Model file for the job. Use its own axes, mm. Coordinates: 2 decimals unless noted, no trailing zeros. Order: outer loops, then holes, each group sorted by start corner. A loop starts at its lowest first (then second) coordinate and runs counter-clockwise, first axis right, second up. Notation, with made-up numbers: (-2.5, 47) - (31.5, 47) arc R37 ccw to (31.5, 83) - close; hole circle Ø7 at (-30.5, -31.5). An arc over 180 degrees is marked (long way). Put each result on its own line as item: value. Start each with the question number.
```python
from build123d import *

# Parameters (mm, degrees)
F0_W     = 60
F0_H     = 60
F1_DEPTH = 10
F2_R     = 4.99999


# Not quite as in the source:
# - a fillet or chamfer is up to 0.001 mm smaller than in the source, because OpenCascade refuses the exact size


with BuildPart() as f1:
    # F0 (on Top) → F1 (new body)
    with BuildSketch(Plane.XY):
        with Locations((1.3857496455, 11.266246149)):
            Rectangle(F0_W, F0_H)
    extrude(amount=F1_DEPTH)

    # F2 (radius 5 in the source; OpenCascade refuses exactly that, so slightly less here)
    f2_edges = [f1.edges().sort_by_distance(p)[0] for p in [
        (-28.61425, 41.266246, 5),
        (-28.61425, -18.733754, 5),
        (-28.61425, 11.266246, 0),
        (-28.61425, 11.266246, 10),
        (31.38575, 41.266246, 5),
        (1.38575, 41.266246, 0),
        (1.38575, 41.266246, 10),
        (31.38575, -18.733754, 5),
        (1.38575, -18.733754, 0),
        (1.38575, -18.733754, 10),
        (31.38575, 11.266246, 0),
        (31.38575, 11.266246, 10),
    ]]
    fillet(f2_edges, radius=F2_R)


solid = f1.part
```
Item 1: Slice it at B-B, the plane z = 1.5. Give the cut face in (x, y).
Item 2: Flat gauge pins, fed straight in: pin 1 Ø6 at (x, z) = (-19, 9) entering from -Y; pin 2 Ø1.5 at (y, z) = (-3.5, 3.5) entering from +X; pin 3 Ø1.5 at (x, z) = (-13, 3) entering from +Y. Where does each tip first touch, or does it go through?
Item 3: Wall check: line 1 along Y through (x, z) = (-14, 4.75); line 2 along Y through (x, z) = (23, 4); line 3 along X through (y, z) = (37, 5.25). Give the ranges that are in metal, low to high.
Here are the results:
1. outline: (-27.18, -13.73) arc R3.57 ccw to (-23.61, -17.3) - (26.39, -17.3) arc R3.57 ccw to (29.96, -13.73) - (29.96, 36.27) arc R3.57 ccw to (26.39, 39.84) - (-23.61, 39.84) arc R3.57 ccw to (-27.18, 36.27) - close
2. pin 1: stops at y = -18.63
2. pin 2: stops at x = 31.33
2. pin 3: stops at y = 41.11
3. line 1: y = -18.73 to 41.26
3. line 2: y = -18.63 to 41.17
3. line 3: x = -28.55 to 31.33
